Could you check a few things on this model? Use its own coordinates, in mm. A direction names the side the tool comes from. Round coordinates to 2 decimals unless told otherwise and drop trailing zeros. Order: outer loops, then holes, each group sorted by start corner. A loop starts at its lowest first (then second) coordinate and runs counter-clockwise, first axis right, second up. Notation, with made-up numbers: (-37.5, 42) -> (-21.5, 42) arc R18 ccw to (-21.5, 48) -> close; hole circle Ø7 at (-12, 87). An arc over 180 degrees is marked (long way). One line per question, with ' | ' between items.
```python
from build123d import *

# Parameters (mm, degrees)
SKETCH_1_W          = 34
SKETCH_1_H          = 35
EXTRUDE_1_DEPTH     = 3
SKETCH_2_W          = 5
SKETCH_2_H          = 5
EXTRUDE_2_DEPTH     = 3
SKETCH_3_R          = 10
EXTRUDE_3_DEPTH     = 3
SKETCH_4_R          = 1.25
CUT_EXTRUDE_1_DEPTH = 3
SKETCH_6_R          = 1.75
CUT_EXTRUDE_6_DEPTH = 1.5
SKETCH_7_R          = 1.5
CUT_EXTRUDE_7_DEPTH = 3


with BuildPart() as part:
    # 草图1 → 凸台-拉伸1 (new body)
    with BuildSketch(Plane.XY):
        Rectangle(SKETCH_1_W, SKETCH_1_H)
    extrude(amount=EXTRUDE_1_DEPTH)

    # 草图2 → 凸台-拉伸2 (add)
    with BuildSketch(Plane.XY.offset(3)):
        with Locations((-19.5, 2.5)):
            Rectangle(SKETCH_2_W, SKETCH_2_H)
        with Locations((-19.5, -2.5)):
            Rectangle(SKETCH_2_W, SKETCH_2_H)
    extrude(amount=-EXTRUDE_2_DEPTH)

    # 草图3 → 凸台-拉伸3 (add)
    with BuildSketch(Plane.ZY.offset(22)):
        with Locations((1.5, 0)):
            Circle(SKETCH_3_R)
    extrude(amount=EXTRUDE_3_DEPTH)

    # 草图4 → 切除-拉伸1 (cut)
    with BuildSketch(Plane.ZY.offset(25)):
        with Locations((1.5, 7)):
            Circle(SKETCH_4_R)
        with Locations((8.5, 0)):
            Circle(SKETCH_4_R)
        with Locations((1.5, -7)):
            Circle(SKETCH_4_R)
        with Locations((-5.5, 0)):
            Circle(SKETCH_4_R)
    extrude(amount=-CUT_EXTRUDE_1_DEPTH, mode=Mode.SUBTRACT)

    # 草图6 → 切除-拉伸6 (cut)
    with BuildSketch(Plane.ZY.offset(25)):
        with Locations((1.5, 0)):
            Circle(SKETCH_6_R)
    extrude(amount=-CUT_EXTRUDE_6_DEPTH, mode=Mode.SUBTRACT)

    # 草图7 → 切除-拉伸7 (cut)
    with BuildSketch(Plane.XY.offset(3)):
        with Locations((10.27515824, 10)):
            Circle(SKETCH_7_R)
        with Locations((10.27515824, -10)):
            Circle(SKETCH_7_R)
        with Locations((-9.593631375, 10)):
            Circle(SKETCH_7_R)
        with Locations((-9.593631375, -10)):
            Circle(SKETCH_7_R)
    extrude(amount=-CUT_EXTRUDE_7_DEPTH, mode=Mode.SUBTRACT)


solid = part.part
```
1. I want a section at A-A on y = 0. List the corners of the cut face in (x, z) for me, and give its area (3 significant figures).
From the geometry:
outline: (-25, -8.5) -> (-22, -8.5) -> (-22, -6.75) -> (-25, -6.75) -> close; (-25, -4.25) -> (-22, -4.25) -> (-22, 0) -> (17, 0) -> (17, 3) -> (-22, 3) -> (-22, 7.25) -> (-25, 7.25) -> (-25, 3.25) -> (-23.5, 3.25) -> (-23.5, -0.25) -> (-25, -0.25) -> close; (-25, 9.75) -> (-22, 9.75) -> (-22, 11.5) -> (-25, 11.5) -> close | area: 157 mm²
2. I want a section at D-D on x = 3. List the corners of the cut face in (y, z) for me.
From the geometry:
outline: (-17.5, 0) -> (17.5, 0) -> (17.5, 3) -> (-17.5, 3) -> close
3. If we mould it in two halves opening along Z, with no side actions, what happens to faces 1 (the face through (17, 0, 1)), 2 (the face through (-23.5, 0, 1)), 3 (the face through (-3, 0, 0))? For each: pulls with the +Z half, pulls with the -Z half, needs draft (parallel to the pull), parting line crosses it, or undercut.
From the geometry:
face 1: needs draft | face 2: undercut | face 3: pulls with the -Z half
4. I want a section at C-C on x = -9. List the corners of the cut face in (y, z) for me, and give its area (3 significant figures).
From the geometry:
outline: (-17.5, 0) -> (-11.38, 0) -> (-11.38, 3) -> (-17.5, 3) -> close; (-8.62, 0) -> (8.62, 0) -> (8.62, 3) -> (-8.62, 3) -> close; (11.38, 0) -> (17.5, 0) -> (17.5, 3) -> (11.38, 3) -> close | area: 88.5 mm²
5. I need wall thicknesses on probe 1 along Y at (x, z) = (-23.15, 1.5); probe 2 along X at (y, z) = (6, 8.25); probe 3 along Z at (x, y) = (-17.5, -4). Which ranges of each line are inside material? Lowest first, please.
From the geometry:
probe 1: y = -10 to -8.25, -5.75 to 5.75, 8.25 to 10 | probe 2: x = -25 to -22 | probe 3: z = 0 to 3
6. I'm going to push flat-ended pins straight in: pin 1 (8 mm diameter, centred on x = 11.5, y = -2, fed in from +Z); pin 2 (4 mm diameter, centred on x = 4, z = -3.5, fed in from +Y) (3 decimals); pin 3 (4 mm diameter, centred on x = 10.28, y = 10, fed in from -Z); pin 4 (2 mm diameter, centred on y = 0, z = 1.5, fed in from -X). Where does each tip first touch, or does it pass through?
From the geometry:
pin 1: stops at z = 3 | pin 2: passes through | pin 3: stops at z = 0 | pin 4: stops at x = -23.5
7. On a 3-axis mill with a long thin cutter (end or side, diameter ignored), from which of +Z, -Z, +X, -X, +Y, -Y can I reach the whole of each face in a straight line? I mean faces 4 (the face through (0, -17.5, 1)), 5 (the face through (-17, 11, 1)), 6 (the face through (-17, -11, 1)), 7 (the face through (-23.52, -8.22, 1.23)). Say none if no direction works.
From the geometry:
face 4: +Z, -Z, +X, -X, -Y | face 5: +Z, -Z, +Y | face 6: +Z, -Z, -Y | face 7: -X
8. I want a section at B-B on z = 2. List the corners of the cut face in (x, y) for me.
From the geometry:
outline: (-25, -9.99) -> (-22, -9.99) -> (-22, -8.15) -> (-25, -8.15) -> close; (-25, -5.85) -> (-22, -5.85) -> (-22, -5) -> (-17, -5) -> (-17, -17.5) -> (17, -17.5) -> (17, 17.5) -> (-17, 17.5) -> (-17, 5) -> (-22, 5) -> (-22, 5.85) -> (-25, 5.85) -> (-25, 1.68) -> (-23.5, 1.68) -> (-23.5, -1.68) -> (-25, -1.68) -> close; (-25, 8.15) -> (-22, 8.15) -> (-22, 9.99) -> (-25, 9.99) -> close; hole circle Ø3 at (-9.59, -10); hole circle Ø3 at (-9.59, 10); hole circle Ø3 at (10.28, -10); hole circle Ø3 at (10.28, 10)
